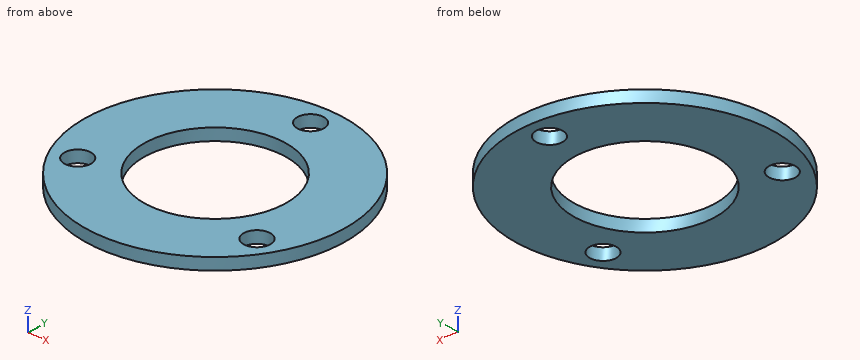
```python
from build123d import *

# Parameters (mm, degrees)
SKETCH1_R               = 22
SKETCH1_R_2             = 12
BOSS_EXTRUDE1_DEPTH     = 1
CUT_EXTRUDE1_DEPTH      = 32.176914536
CUT_EXTRUDE1_DEPTH_BACK = 32.176914536
SKETCH2_R               = 2.25


with BuildPart() as part:
    # Sketch1 → Boss-Extrude1 (new, symmetric)
    with BuildSketch(Plane.XY):
        Circle(SKETCH1_R)
        Circle(SKETCH1_R_2, mode=Mode.SUBTRACT)
    extrude(amount=BOSS_EXTRUDE1_DEPTH, both=True)

    # Sketch2 → Cut-Extrude1 (cut, two sides: drawn at the far end of the back side and taken through both)
    with BuildSketch(Plane.XY.offset(1).offset(-CUT_EXTRUDE1_DEPTH_BACK)):
        with Locations((0, 18)):
            Circle(SKETCH2_R)
        with Locations((15.588457268, -9)):
            Circle(SKETCH2_R)
        with Locations((-15.588457268, -9)):
            Circle(SKETCH2_R)
    extrude(amount=CUT_EXTRUDE1_DEPTH + CUT_EXTRUDE1_DEPTH_BACK, mode=Mode.SUBTRACT)


solid = part.part
```
Could you check a few things on this model? Use its own coordinates, in mm. Round coordinates to 2 decimals unless told otherwise and drop trailing zeros. Loops run counter-clockwise (first coordinate to the right, second up) from the corner with the lowest first, then second, coordinate; pieces in that order, holes last.
Q1. I want a section at A-A (y = 0). Write out the boundary of the cut face in (x, z), and give its area (3 significant figures).
Q2. I want a section at C-C (x = -17). Write out the boundary of the cut face in (y, z), and give its area (3 significant figures).
Q3. I want a section at D-D (z = -0.55). Write out the boundary of the cut face in (x, y).
Q4. Please list where these lines run through material, in increasing order: L1, parallel to Y at x = 0, z = 0.5; L2, parallel to X at y = -10.5, z = -0.45; L3, parallel to X at y = -9, z = -0.1.
Q5. I want a section at B-B (x = 0). Write out the boundary of the cut face in (y, z), and give its area (3 significant figures).
Answer below:
1. outline: (-22, -1) - (-12, -1) - (-12, 1) - (-22, 1) - close; (12, -1) - (22, -1) - (22, 1) - (12, 1) - close
1. area: 40.0 mm2
2. outline: (-13.96, -1) - (-10.75, -1) - (-10.75, 1) - (-13.96, 1) - close; (-7.25, -1) - (13.96, -1) - (13.96, 1) - (-7.25, 1) - close
2. area: 48.8 mm2
3. outline: circle Ø44 at (0, 0); hole circle Ø4.5 at (-15.59, -9); hole circle Ø24 at (0, 0); hole circle Ø4.5 at (0, 18); hole circle Ø4.5 at (15.59, -9)
4. L1: y = -22 to -12, 12 to 15.75, 20.25 to 22
4. L2: x = -19.33 to -17.27, -13.91 to -5.81, 5.81 to 13.91, 17.27 to 19.33
4. L3: x = -20.07 to -17.84, -13.34 to -7.94, 7.94 to 13.34, 17.84 to 20.07
5. outline: (-22, -1) - (-12, -1) - (-12, 1) - (-22, 1) - close; (12, -1) - (15.75, -1) - (15.75, 1) - (12, 1) - close; (20.25, -1) - (22, -1) - (22, 1) - (20.25, 1) - close
5. area: 31.0 mm2
